Autodesk Inventor part; units mm, degrees
ref_plane "YZ Plane" through (0, 0, 0) normal (1, 0, 0) x (0, 1, 0)
ref_plane "XZ Plane" through (0, 0, 0) normal (0, 1, 0) x (-1, 0, 0)
ref_plane "XY Plane" through (0, 0, 0) normal (0, 0, 1) x (1, 0, 0)
sketch "Эскиз1" plane through (0, 0, 0) normal (0, 1, 0) x (-1, 0, 0)
  circle A0 centre (0, 0) radius 7.5
  dimension "d0" = 15
extrude "Выдавливание1" add sketch "Эскиз1" along normal blind 1.5
sketch "Эскиз2" plane through (0, 1.5, 0) normal (0, 1, 0) x (1, 0, 0)
  circle A0 centre (0, 0) radius 7.5
  circle A1 centre (0, 0) radius 4.9
  dimension "d3" = 9.8
extrude "Выдавливание2" add sketch "Эскиз2" along normal blind 7 contours A1
sketch "Эскиз4" plane through (0, 8.5, 0) normal (0, 1, 0) x (1, 0, 0)
  circle A0 centre (0, 0) radius 4.9
  circle A1 centre (0, 0) radius 3.3
  dimension "d9" = 6.6
extrude "Выдавливание4" cut sketch "Эскиз4" against normal through all contours A1
properties part number "Шайба_Уплотнитель"
CAD build for the part. Positions are in the model's coordinates, mm. A direction names the side the tool comes from. Round coordinates to 2 decimals unless told otherwise and drop trailing zeros. Order: outer loops, then holes, each group sorted by start corner. A loop starts at its lowest first (then second) coordinate and runs counter-clockwise, first axis right, second up. Notation, with made-up numbers: (68.5, -22.5) -> (102.5, -22.5) arc R23 ccw to (102.5, 10.5) -> close; hole circle Ø6 at (-2, -13.75). An arc over 180 degrees is marked (long way). One line per question, with ' | ' between items.
Q1. Slice it at C-C (y = 4.5). Write the cut outline in (x, z).
Completed:
outline: circle Ø9.8 at (0, 0); hole circle Ø6.6 at (0, 0)
Q2. Probe probe 1 along Z at (x, y) = (0, 4); probe 2 along Y at (x, z) = (5, -4). List the from-to ranges inside material, lowest first.
Completed:
probe 1: z = -4.9 to -3.3, 3.3 to 4.9 | probe 2: y = 0 to 1.5
Q3. Drop flat-ended pins along their axis: pin 1 (5 mm diameter, centred on x = -5, y = 3.5, fed in from -Z); pin 2 (5 mm diameter, centred on x = 4.5, y = 5, fed in from -Z); pin 3 (2 mm diameter, centred on x = 5.5, y = 7.5, fed in from -Z). Give the stop position or say it passes through.
Completed:
pin 1: stops at z = -6.63 | pin 2: stops at z = -4.47 | pin 3: stops at z = -1.94
Q4. Which spindle directions (+Z, -Z, +X, -X, +Y, -Y) get a long thin tool onto all of the face, cutting with end or side? Do faces 1 (the cylindrical face through (7.493, 0.74, -0.33)), 2 (the flat face through (-2, 1.5, -5)). Say none if no direction does.
Completed:
face 1: +Y, -Y | face 2: +Y
Q5. Slice it at D-D (z = -3.75). Write the cut outline in (x, y), then the cut area to 3 significant figures.
Completed:
outline: (-6.5, 0) -> (6.5, 0) -> (6.5, 1.5) -> (3.15, 1.5) -> (3.15, 8.5) -> (-3.15, 8.5) -> (-3.15, 1.5) -> (-6.5, 1.5) -> close | area: 63.6 mm^2
Q6. Slice it at A-A (z = 0). Write the cut outline in (x, y).
Completed:
outline: (-7.5, 0) -> (-3.3, 0) -> (-3.3, 8.5) -> (-4.9, 8.5) -> (-4.9, 1.5) -> (-7.5, 1.5) -> close; (3.3, 0) -> (7.5, 0) -> (7.5, 1.5) -> (4.9, 1.5) -> (4.9, 8.5) -> (3.3, 8.5) -> close
Q7. Two-plate mould, pull along Z, no slides. Class faces 3 (the cylindrical face through (-2.43, 4.31, -2.23)), 4 (the cylindrical face through (-1.062, 4.951, -4.783)), 5 (the flat face through (-2, 0, -3)): released by +Z, released by -Z, zero draft, split by the parting line, or undercut.
Completed:
face 3: undercut | face 4: split by the parting line | face 5: zero draft
Q8. Slice it at B-B (x = -1.5). Write the cut outline in (y, z).
Completed:
outline: (0, -7.35) -> (1.5, -7.35) -> (1.5, -4.66) -> (8.5, -4.66) -> (8.5, -2.94) -> (0, -2.94) -> close; (0, 2.94) -> (8.5, 2.94) -> (8.5, 4.66) -> (1.5, 4.66) -> (1.5, 7.35) -> (0, 7.35) -> close
